Work out the finished part from the listing and answer in its coordinate system (mm). Give positions to 0.01 mm unless a question says otherwise; leave off trailing zeros. Loops run counter-clockwise (first coordinate to the right, second up) from the corner with the lowest first, then second, coordinate; pieces in that order, holes last.
```python
from build123d import *

# Parameters (mm, degrees)
F0_W     = 457.2
F0_H     = 63.5
F1_DEPTH = 19.05
F3_D     = 6.35


with BuildPart() as f1:
    # F0 (on Front) → F1 (new body)
    with BuildSketch(Plane.XZ):
        with Locations((228.6, 0)):
            Rectangle(F0_W, F0_H)
        with BuildLine():
            ThreePointArc((0, 31.75), (-31.75, 0), (0, -31.75))
            Line((0, -31.75), (0, 31.75))
        make_face()
        with BuildLine():
            Line((457.2, 31.75), (457.2, -31.75))
            ThreePointArc((457.2, -31.75), (488.95, 0), (457.2, 31.75))
        make_face()
    extrude(amount=F1_DEPTH)

    # F3 (through all)
    with Locations(Plane(origin=(0, 0, 0), x_dir=(-1, 0, 0), z_dir=(0, 1, 0))):
        with Locations((-457.2, 0), (0, 0), (-228.6, 0)):
            Hole(F3_D / 2)


solid = f1.part
```
Q1. Section C-C on z = 21 is taken. Give the vertices of the cut face in (x, y), plus the area to 3 significant figures.
Q2. Consider line 1 along Z through (x, y) = (0, -12.75) (3 decimals); line 2 along X through (y, z) = (-3.25, -24). Determine where each line is inside the solid, lowest interval first.
Q3. Section B-B on z = -20 is taken. Give the vertices of the cut face in (x, y), plus the area to 3 significant figures.
Q4. Section A-A on y = -14.5 is taken. Give the vertices of the cut face in (x, z) (3 decimals).
Q5. Given pin 1 (2 mm diameter, centred on y = -14, z = 0, fed in from +X); pin 2 (6 mm diameter, centred on y = -11, z = -9, fed in from +X); pin 3 (2 mm diameter, centred on y = -10, z = 6, fed in from +X), each flat-ended and moving along its own axis, determine where each tip first touches the part or whether it passes through.
Check result:
1. outline: (-23.81, -19.05) - (481.01, -19.05) - (481.01, 0) - (-23.81, 0) - close
1. area: 9,620 mm2
2. line 1: z = -31.75 to -3.175, 3.175 to 31.75
2. line 2: x = -20.79 to 477.99
3. outline: (-24.66, -19.05) - (481.86, -19.05) - (481.86, 0) - (-24.66, 0) - close
3. area: 9,650 mm2
4. outline: (0, -31.75) - (457.2, -31.75) arc R31.75 ccw to (457.2, 31.75) - (0, 31.75) arc R31.75 ccw to start; hole circle Ø6.35 at (0, 0); hole circle Ø6.35 at (228.6, 0); hole circle Ø6.35 at (457.2, 0)
5. pin 1: stops at x = 488.95
5. pin 2: stops at x = 488.38
5. pin 3: stops at x = 488.55
